Autodesk Fusion 360 part; units mm, degrees
sketch "Sketch1" plane through (0, 0, 0) normal (0, 1, 0) x (1, 0, 0)
  line L0 (-137.3579, 25) -> (62.6421, 25)
  line L1 (62.6421, 25) -> (62.6421, -65)
  line L2 (-137.3579, -65) -> (-137.3579, 25)
  line L3 (-97.3579, -65) -> (-97.3579, -25)
  line L4 (-97.3579, -25) -> (22.6421, -25)
  line L5 (22.6421, -25) -> (22.6421, -65)
  line L6 (62.6421, -65) -> (22.6421, -65)
  line L7 (-97.3579, -65) -> (-137.3579, -65)
  dimension "d1" = 200
  dimension "d2" = 90
  dimension "d8" = 50
extrude "Extrude1" add sketch "Sketch1" along normal blind 40
fillet "Fillet1" radius 10 6 edges at (-137.3579, 20, 65) (-97.3579, 20, 65) (-97.3579, 20, 25) (22.6421, 20, 25) (22.6421, 20, 65) (62.6421, 20, 65)
fillet "Fillet2" radius 15 2 edges at (-137.3579, 20, -25) (62.6421, 20, -25)
sketch "Sketch2" plane through (0, 0, 0) normal (0, -1, 0) x (1, 0, 0)
  arc A0 (47.6421, -25) -> (62.6421, -10) centre (47.6421, -10) ccw
  line L0 (62.6421, -10) -> (62.6421, 55)
  arc A1 (62.6421, 55) -> (52.6421, 65) centre (52.6421, 55) ccw
  line L1 (52.6421, 65) -> (32.6421, 65)
  arc A2 (32.6421, 65) -> (22.6421, 55) centre (32.6421, 55) ccw
  line L2 (22.6421, 55) -> (22.6421, 35)
  arc A3 (12.6421, 25) -> (22.6421, 35) centre (12.6421, 35) ccw
  line L3 (12.6421, 25) -> (-87.3579, 25)
  arc A4 (-97.3579, 35) -> (-87.3579, 25) centre (-87.3579, 35) ccw
  line L4 (-97.3579, 35) -> (-97.3579, 55)
  arc A5 (-97.3579, 55) -> (-107.3579, 65) centre (-107.3579, 55) ccw
  line L5 (-107.3579, 65) -> (-127.3579, 65)
  arc A6 (-127.3579, 65) -> (-137.3579, 55) centre (-127.3579, 55) ccw
  line L6 (-137.3579, 55) -> (-137.3579, -10)
  arc A7 (-137.3579, -10) -> (-122.3579, -25) centre (-122.3579, -10) ccw
  line L7 (-122.3579, -25) -> (47.6421, -25)
  circle A8 centre (-122.3579, -10) radius 7.5
  circle A9 centre (47.6421, -10) radius 7.5
  dimension "d13" = 15
  dimension "d14" = 15
extrude "Extrude2" cut sketch "Sketch2" against normal blind 40 contours A8 | A9
properties part number "Tutorial Part 1"
Geometry: final body of the model. Coordinates: model frame, mm. A direction names the side the tool comes from. Round coordinates to 2 decimals unless told otherwise and drop trailing zeros. Loops run counter-clockwise (first coordinate to the right, second up) from the corner with the lowest first, then second, coordinate; pieces in that order, holes last. Notation, with made-up numbers: (-32, -8) -> (27, -8) arc R24 ccw to (27, 6) -> close; hole circle Ø5 at (-23, 9.25). An arc over 180 degrees is marked (long way). Use one line per item in the form item = value. Start each with the question number.
1) Section C-C on z = 44.5. Output: boundary loops of the cut face in (x, y).
2) Section D-D on x = -49. Output: boundary loops of the cut face in (y, z), then the cut area to 3 significant figures.
3) Draft query along Z for faces 3 (the cylindrical face through (25.5, 20.3, 62)), 4 (the cylindrical face through (40.15, 19.72, -9.67)), 5 (the cylindrical face through (-115.204, 19.72, -7.747)), 6 (the flat face through (-39, 0, 9)). Return one class per face: released by +Z, released by -Z, zero draft, split by the parting line, or undercut.
4) Access query for faces 1 (the cylindrical face through (-100.365, 20.28, 62.148)), 2 (the flat face through (62.642, 20, 22)). Directions: +Z, -Z, +X, -X, +Y, -Y. A direction counts if a zero-diameter tool reaches every point of the face in a straight line with its end or side. Return the directions, or none.
5) Line query: L1, parallel to X at y = 36, z = -15; L2, parallel to X at y = 33, z = 34.5; L3, parallel to Z at x = 8, y = 18.5. Output: solid intervals per line, ascending.
6) Section A-A on y = 6. Output: boundary loops of the cut face in (x, z), then the cut area to 3 significant figures.
7) First-contact query: P1, Ø5, axis at y = 25.5, z = -15, coming from the +X side; P2, Ø1.5, axis at y = 9, z = -15, coming from the +X side; P3, Ø9, axis at x = -122.36, z = -10, coming from the -Y side. Flat tips, straight axial feed; report the tip coordinate or a pass-through.
8) Section B-B on z = 28. Output: boundary loops of the cut face in (x, y), then the cut area to 3 significant figures.
Response:
q1.outline = (-137.36, 0) -> (-97.36, 0) -> (-97.36, 40) -> (-137.36, 40) -> close; (22.64, 0) -> (62.64, 0) -> (62.64, 40) -> (22.64, 40) -> close
q2.outline = (0, -25) -> (40, -25) -> (40, 25) -> (0, 25) -> close
q2.area = 2,000 mm^2
q3.face_3 = released by +Z
q3.face_4 = undercut
q3.face_5 = undercut
q3.face_6 = zero draft
q4.face_1 = +Z, +Y, -Y
q4.face_2 = +Z, -Z, +X, +Y, -Y
q5.L1 = -136.5 to -127.95, -116.77 to 42.05, 53.23 to 61.78
q5.L2 = -137.36 to -97.35, 22.63 to 62.64
q5.L3 = -25 to 25
q6.outline = (-137.36, -10) arc R15 ccw to (-122.36, -25) -> (47.64, -25) arc R15 ccw to (62.64, -10) -> (62.64, 55) arc R10 ccw to (52.64, 65) -> (32.64, 65) arc R10 ccw to (22.64, 55) -> (22.64, 35) arc R10 cw to (12.64, 25) -> (-87.36, 25) arc R10 cw to (-97.36, 35) -> (-97.36, 55) arc R10 ccw to (-107.36, 65) -> (-127.36, 65) arc R10 ccw to (-137.36, 55) -> close; hole circle Ø15 at (-122.36, -10); hole circle Ø15 at (47.64, -10)
q6.area = 12,700 mm^2
q7.P1 = 62.43
q7.P2 = 62.03
q7.P3 = through
q8.outline = (-137.36, 0) -> (-94.5, 0) -> (-94.5, 40) -> (-137.36, 40) -> close; (19.78, 0) -> (62.64, 0) -> (62.64, 40) -> (19.78, 40) -> close
q8.area = 3,430 mm^2
